Part model, mm, in its own coordinate system. Face numbers are marked on the shaded views. A direction names the side the tool comes from. Coordinates: 2 decimals unless noted, no trailing zeros. Loops run counter-clockwise (first coordinate to the right, second up) from the corner with the lowest first, then second, coordinate; pieces in that order, holes last. Notation, with made-up numbers: M 70.25,39 L 103.25,39 A25 cw 103.25,56 Z; hole C 9,-2.5 d1. An arc over 180 degrees is marked long. Use a Markdown table: item, result. Add a question column.
1) Band-saw the part on A-A (y = 32). List the corners of the cut face in (x, z).
2) Pin check, flat tips, straight feed: pin 1 Ø5 at (x, z) = (-3, 4) entering from +Y; pin 2 Ø3 at (x, z) = (11.75, 5) entering from +Y; pin 3 Ø1.5 at (y, z) = (7, 2.5) entering from +X. Stop position of each tip, or through.
3) Band-saw the part on D-D (x = 11.75). List the corners of the cut face in (y, z), plus the area to 3 significant figures.
4) Tool access for the marked faces 1 and 2: list every direction of +Z, -Z, +X, -X, +Y, -Y with a clear straight run to the whole face (end or side of a thin tool).
5) Wall check: probe 1 along X at (y, z) = (34, 6.25); probe 2 along X at (y, z) = (1.25, 5); probe 3 along X at (y, z) = (2, 5). Give the ranges that are in metal, low to high. Write a range as from..to.
6) Pull direction X, two halves, no side cores. Call the marked faces 3, 4 and 5: released by +X, released by -X, zero draft, split by the parting line, or undercut.
7) Band-saw the part on C-C (x = -28). List the corners of the cut face in (y, z).
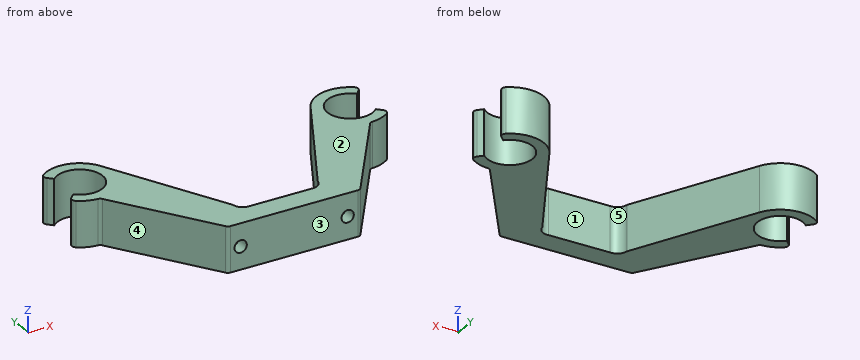
from build123d import *

# Parameters (mm, degrees)
BOSS_EXTRUDE2_DEPTH = 10
SKETCH2_R           = 5
CUT_EXTRUDE1_DEPTH  = 10
SKETCH3_R           = 1.35
CUT_EXTRUDE2_DEPTH  = 3
FILLET1_R           = 1
FILLET2_R           = 1


with BuildPart() as part:
    # Sketch1 → Boss-Extrude2 (new body)
    with BuildSketch(Plane.XY):
        with BuildLine():
            Line((14.5, 0), (-14.5, 0))
            Line((-14.5, 0), (-29.68, 22))
            ThreePointArc((-29.68, 22), (-32.550125743, 22.570903506), (-34.983300859, 24.196699141))
            Line((-34.983300859, 24.196699141), (-29.68, 29.5))
            Line((-29.68, 29.5), (-34.983300859, 34.803300859))
            ThreePointArc((-34.983300859, 34.803300859), (-28.562836183, 36.916329618), (-23.049751963, 33.005682668))
            Line((-23.049751963, 33.005682668), (-9.299486441, 7))
            ThreePointArc((-9.299486441, 7), (-8.438956783, 5.47198407), (-6.75, 5))
            Line((-6.75, 5), (6.75, 5))
            ThreePointArc((6.75, 5), (8.438956783, 5.47198407), (9.299486441, 7))
            Line((9.299486441, 7), (23.049751963, 33.005682668))
            ThreePointArc((23.049751963, 33.005682668), (28.562836183, 36.916329618), (34.983300859, 34.803300859))
            Line((34.983300859, 34.803300859), (29.68, 29.5))
            Line((29.68, 29.5), (34.983300859, 24.196699141))
            ThreePointArc((34.983300859, 24.196699141), (32.550125743, 22.570903506), (29.68, 22))
            Line((29.68, 22), (14.5, 0))
        make_face()
    extrude(amount=BOSS_EXTRUDE2_DEPTH)

    # Sketch2 → Cut-Extrude1 (cut)
    with BuildSketch(Plane.XY.offset(10)):
        with Locations((-29.68, 29.5)):
            Circle(SKETCH2_R)
        with Locations((29.68, 29.5)):
            Circle(SKETCH2_R)
    extrude(amount=-CUT_EXTRUDE1_DEPTH, mode=Mode.SUBTRACT)

    # Sketch3 → Cut-Extrude2 (cut)
    with BuildSketch(Plane.XZ):
        with Locations(Location((-11.75, 5, 0), (0, 0, 270))):
            Circle(SKETCH3_R)
        with Locations(Location((11.75, 5, 0), (0, 0, 270))):
            Circle(SKETCH3_R)
    extrude(amount=-CUT_EXTRUDE2_DEPTH, mode=Mode.SUBTRACT)

    # Fillet1
    fillet1_edges = [part.edges().sort_by_distance(p)[0] for p in [
        (-34.983300859, 24.196699141, 5),
        (-34.983300859, 34.803300859, 5),
    ]]
    fillet(fillet1_edges, radius=FILLET1_R)

    # Fillet2
    fillet2_edges = [part.edges().sort_by_distance(p)[0] for p in [
        (-29.68, 22, 5),
        (34.983300859, 34.803300859, 5),
        (34.983300859, 24.196699141, 5),
        (29.68, 22, 5),
        (14.5, 0, 5),
        (-14.5, 0, 5),
    ]]
    fillet(fillet2_edges, radius=FILLET2_R)


solid = part.part
Entries:
| question | item | result |
|---|---|---|
| 1 | outline | M -25.35,0 L -22.52,0 L -22.52,10 L -25.35,10 Z; M 22.52,0 L 25.35,0 L 25.35,10 L 22.52,10 Z |
| 2 | pin 1 | y = 5 |
| 2 | pin 2 | y = 14.47 |
| 2 | pin 3 | x = 19.85 |
| 3 | outline | M 0,0 L 11.63,0 L 11.63,10 L 0,10 L 0,6.35 L 3,6.35 L 3,3.65 L 0,3.65 Z |
| 3 | area | 108 mm2 |
| 4 | face 1 | +Z, -Z, +Y |
| 4 | face 2 | +Z, +X, -X, +Y, -Y |
| 5 | probe 1 | -34.18..-31.86, -27.5..-23.68, 23.68..27.5, 31.86..34.18 |
| 5 | probe 2 | -15.36..-13.1, -10.4..10.4, 13.1..15.36 |
| 5 | probe 3 | -15.88..-13.1, -10.4..10.4, 13.1..15.88 |
| 6 | face 3 | zero draft |
| 6 | face 4 | released by -X |
| 6 | face 5 | undercut |
| 7 | outline | M 19.57,0 L 24.79,0 L 24.79,10 L 19.57,10 Z; M 34.21,0 L 36.81,0 L 36.81,10 L 34.21,10 Z |
